Autodesk Inventor part; units mm, degrees
ref_plane "YZ Plane" through (0, 0, 0) normal (1, 0, 0) x (0, 1, 0)
ref_plane "XZ Plane" through (0, 0, 0) normal (0, 1, 0) x (-1, 0, 0)
ref_plane "XY Plane" through (0, 0, 0) normal (0, 0, 1) x (1, 0, 0)
sketch "Sketch1" plane through (0, 0, 0) normal (0, 0, 1) x (1, 0, 0)
  circle A0 centre (0, 0) radius 125
  circle A1 centre (0, 0) radius 164.5
  dimension "d0" = 39.5
  dimension "d1" = 250
extrude "Extrusion1" add sketch "Sketch1" along normal blind 41
sketch "Sketch2" plane through (0, 0, 41) normal (0, 0, 1) x (1, 0, 0)
  circle A0 centre (0, 0) radius 164.5 construction
  circle A1 centre (0, 0) radius 125 construction
  line L0 (0, 164.5) -> (0, 125) construction
  circle A2 centre (0, 144.75) radius 6.25
  dimension "d4" = 12.5
extrude "Extrusion2" cut sketch "Sketch2" against normal through all
sketch "Sketch3" plane through (0, 0, 41) normal (0, 0, 1) x (1, 0, 0)
  circle A0 centre (0, 144.75) radius 6.25
  circle A1 centre (0, 144.75) radius 13.75
  point P0 (0, 0)
  dimension "d10" = 27.5
extrude "Extrusion3" cut sketch "Sketch3" against normal blind 11
pattern_circular "Circular Pattern1" count 8 over 360 about axis through (0, 0, 0) along (0, 0, 1) of "Extrusion2", "Extrusion3"
sketch "Sketch4" plane through (0, 0, 0) normal (0, 0, -1) x (-1, 0, 0)
  circle A0 centre (0, 0) radius 164.5
  circle A1 centre (0, 0) radius 169.5
  dimension "d13" = 5
extrude "Extrusion4" add sketch "Sketch4" against normal blind 10
sketch "Sketch5" plane through (0, 0, 0) normal (1, 0, 0) x (0, 1, 0)
  line L0 (164.5, 10) -> (-164.5, 10)
  line L1 (164.5, 41) -> (-164.5, 41)
  line L2 (169.5, 10) -> (-169.5, 10)
  line L3 (-169.5, 0) -> (169.5, 0)
  line L4 (164.5, 41) -> (164.5, 10)
  line L5 (164.5, 10) -> (164.5, 41)
  line L6 (169.5, 10) -> (169.5, 0)
  line L7 (-164.5, 41) -> (-164.5, 10)
  line L8 (-169.5, 10) -> (-169.5, 0)
  line L9 (-164.5, 22) -> (164.5, 22)
  point P0 (0, 0)
  point P1 (164.5, 22)
  dimension "d16" = 19
  dimension "d17" = 41
extrude "Extrusion5" cut sketch "Sketch5" along normal through all both and the other way through all contours L9 L7 L1 L4
equation "\"d1\" = Вал_ось_диаметр_НОС"
equation "\"BendRadius\" = Thickness"
equation "\"BendReliefWidth\" = Thickness"
equation "\"BendReliefDepth\" = 0.5 * Thickness"
equation "\"CornerReliefSize\" = 4 * Thickness"
equation "\"MinimumRemnant\" = 2 * Thickness"
equation "\"TransitionRadius\" = BendRadius"
equation "\"JacobiRadiusSize\" = BendRadius"
equation "\"GapSize\" = Thickness"
properties part number "ДМФ 01 31.1 Барабан Опорное кольцо НОС"
Model file for the job. Use its own axes, mm. A direction names the side the tool comes from. Coordinates: 2 decimals unless noted, no trailing zeros. Write each loop counter-clockwise with the first axis right and the second up, starting at its lowest first coordinate (ties: lowest second). Pieces come first, ordered by that corner, then holes. Notation, with made-up numbers: (77.5, -37.75) -> (115.5, -37.75) arc R19 ccw to (115.5, -24.75) -> close; hole circle Ø6 at (60, 45.25). An arc over 180 degrees is marked (long way). One line per item, written item: value. Start each with the question number.
1) Slice it at C-C on x = 144.75. Write the cut outline in (y, z).
2) Slice it at A-A on x = 0. Write the cut outline in (y, z), then the cut area to 3 significant figures.
3) Pull direction X, two halves, no side cores. Call faces 1 (the face through (89, 89, 0)), 2 (the face through (-35.66, 160.59, 15.92)), 3 (the face through (98.13, 106.96, 11.15)): +X half, -X half, draft (parallel to the pull), parting line (faces both ways), or undercut.
4) Slice it at B-B on y = 85. Write the cut outline in (x, z), then the cut area to 3 significant figures.
5) Probe probe 1 along Y at (x, z) = (0, 16.75); probe 2 along Y at (x, z) = (0, 5). List the from-to ranges inside material, lowest first.
6) Which spindle directions (+Z, -Z, +X, -X, +Y, -Y) get a long thin tool onto all of the face, cutting with end or side? Do faces 4 (the face through (106.96, -98.13, 11.15)), 5 (the face through (89, 139, 10)). Say none if no direction does.
7) Slice it at D-D on z = 18.25. Count the separate pieces of the cut face and the enclosed holes in it, then the cut area to 3 significant figures.
8) Flat gauge pins, fed straight in: pin 1 Ø11 at (x, y) = (-102.35, 102.35) entering from -Z; pin 2 Ø5 at (y, z) = (23.5, 17.5) entering from -X; pin 3 Ø12 at (x, z) = (-81.5, 19) entering from +Y; pin 4 Ø2 at (y, z) = (135, 17.5) entering from -X. Where does each tip first touch, or does it go through?
Answers follow:
1. outline: (-88.19, 0) -> (-6.25, 0) -> (-6.25, 22) -> (-78.15, 22) -> (-78.15, 10) -> (-88.19, 10) -> close; (6.25, 0) -> (88.19, 0) -> (88.19, 10) -> (78.15, 10) -> (78.15, 22) -> (6.25, 22) -> close
2. outline: (-169.5, 0) -> (-151, 0) -> (-151, 22) -> (-164.5, 22) -> (-164.5, 10) -> (-169.5, 10) -> close; (-138.5, 0) -> (-125, 0) -> (-125, 22) -> (-138.5, 22) -> close; (125, 0) -> (138.5, 0) -> (138.5, 22) -> (125, 22) -> close; (151, 0) -> (169.5, 0) -> (169.5, 10) -> (164.5, 10) -> (164.5, 22) -> (151, 22) -> close
2. area: 1,290 mm2
3. face 1: draft
3. face 2: parting line
3. face 3: undercut
4. outline: (-146.65, 0) -> (-91.65, 0) -> (-91.65, 22) -> (-140.84, 22) -> (-140.84, 10) -> (-146.65, 10) -> close; (91.65, 0) -> (146.65, 0) -> (146.65, 10) -> (140.84, 10) -> (140.84, 22) -> (91.65, 22) -> close
4. area: 2,280 mm2
5. probe 1: -164.5 to -151, -138.5 to -125, 125 to 138.5, 151 to 164.5
5. probe 2: -169.5 to -151, -138.5 to -125, 125 to 138.5, 151 to 169.5
6. face 4: +Z, -Z
6. face 5: +Z
7. separate pieces: 1
7. enclosed holes: 9
7. area: 34,900 mm2
8. pin 1: through
8. pin 2: x = -163.15
8. pin 3: y = 146.15
8. pin 4: x = -95.42
